from build123d import *

# Parameters (mm, degrees)
BOSS_EXTRUDE1_DEPTH   = 4
M4X0_7_TAPPED_HOLE1_D = 3.3


with BuildPart() as part:
    # Sketch1 → Boss-Extrude1 (new body)
    with BuildSketch(Plane.XY):
        Polygon((-2.886751346, 5), (-5.773502692, 0), (-2.886751346, -5), (2.886751346, -5), (5.773502692, 0), (2.886751346, 5), align=None)
    extrude(amount=BOSS_EXTRUDE1_DEPTH)

    # M4x0.7 Tapped Hole1 (through all)
    with Locations(Plane(origin=(0, 0, 0), x_dir=(-1, 0, 0), z_dir=(0, 0, -1))):
        with Locations((0, 0)):
            Hole(M4X0_7_TAPPED_HOLE1_D / 2)

    # Sketch3 → Cut-Revolve3 (revolve, cut)
    with BuildSketch(Plane(origin=(0, 0, 0), x_dir=(1, 0, 0), z_dir=(0, 1, 0))):
        Polygon((6.057291813, -1.351831913), (1.65, -4), (6.057291813, -4), align=None)
    revolve(axis=Axis((0, 0, 4), (0, 0, 1)), mode=Mode.SUBTRACT)

    # Sketch5 → Cut-Revolve4 (revolve, cut)
    with BuildSketch(Plane(origin=(0, 0, 0), x_dir=(1, 0, 0), z_dir=(0, 1, 0))):
        Polygon((5.023502692, 0), (5.773502692, -0.433012702), (5.773502692, 0), align=None)
    revolve(axis=Axis((0, 0, 0), (0, 0, 1)), mode=Mode.SUBTRACT)


solid = part.part
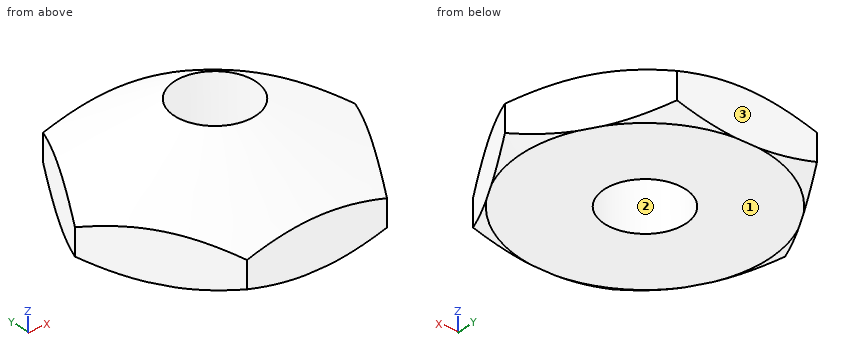
Check sheet for the modelled part. Datum: model origin and axes. Units: mm. Face numbers are marked on the shaded views. Round coordinates to 2 decimals unless told otherwise and drop trailing zeros. Loops run counter-clockwise (first coordinate to the right, second up) from the corner with the lowest first, then second, coordinate; pieces in that order, holes last.
1. Scan lines: probe 1 along Y at (x, z) = (0, 1.25); probe 2 along X at (y, z) = (2.25, 2.95); probe 3 along X at (y, z) = (1.5, 1.2). Record each from-to range of solid material in increasing order.
2. Gauge pin test, flat ends, axial feed: pin 1 Ø1.5 at (y, z) = (2.5, 1.5) entering from -X; pin 2 Ø6 at (x, y) = (-2.5, 3) entering from +Z; pin 3 Ø2 at (x, y) = (0, 0) entering from +Z. Record the tip position at first contact, or that the pin passes through.
3. Sectioned sample at A-A on x = 0. Record the boundary of the cut face in (y, z), and give its area (3 significant figures).
4. Sectioned sample at C-C on z = 3.1. Record the boundary of the cut face in (x, y), and give its area (3 significant figures).
5. Sectioned sample at D-D on z = 2.45. Record the boundary of the cut face in (x, y), and give its area (3 significant figures).
6. Sectioned sample at B-B on z = 1.1. Record the boundary of the cut face in (x, y).
7. Mould release check, pull along Y, two halves, no side actions. Record for the marked faces 1, 2 and 3: released by +Y, released by -Y, zero draft, split by the parting line, or undercut.
Recorded:
1. probe 1: y = -5 to -1.65, 1.65 to 5
1. probe 2: x = -2.55 to 2.55
1. probe 3: x = -4.91 to -0.69, 0.69 to 4.91
2. pin 1: stops at x = -4.76
2. pin 2: stops at z = 4
2. pin 3: passes through
3. outline: (-5, 0) - (-1.65, 0) - (-1.65, 4) - (-5, 1.99) - close; (1.65, 0) - (5, 0) - (5, 1.99) - (1.65, 4) - close
3. area: 20.1 mm2
4. outline: circle Ø6.3 at (0, 0); hole circle Ø3.3 at (0, 0)
4. area: 22.6 mm2
5. outline: circle Ø8.46 at (0, 0); hole circle Ø3.3 at (0, 0)
5. area: 47.6 mm2
6. outline: (-5.77, 0) - (-2.89, -5) - (2.89, -5) - (5.77, 0) - (2.89, 5) - (-2.89, 5) - close; hole circle Ø3.3 at (0, 0)
7. face 1: zero draft
7. face 2: undercut
7. face 3: released by +Y
